Can you work these out from the model? Positions are in its coordinate system, mm. A direction names the side the tool comes from. Round coordinates to 2 decimals unless told otherwise and drop trailing zeros. Loops run counter-clockwise (first coordinate to the right, second up) from the corner with the lowest first, then second, coordinate; pieces in that order, holes last. Notation, with made-up numbers: M -38,48 L -10,48 A26 cw -10,66 Z; hole C 30.25,80 d1. An arc over 180 degrees is marked long. Return JSON: item names as keys, results as strings.
```python
from build123d import *

# Parameters (mm, degrees)
SKETCH3_W            = 88.9
SKETCH3_H            = 88.9
BOSS_EXTRUDE2_DEPTH  = 50.8
SKETCH13_R           = 4.25
CUT_EXTRUDE4_DEPTH   = 102
SKETCH30_W           = 88.9
SKETCH30_H           = 88.9
SKETCH30_W_2         = 60
SKETCH30_H_2         = 60
BOSS_EXTRUDE8_DEPTH  = 110
SKETCH31_W           = 15
SKETCH31_H           = 15
SKETCH31_R           = 2.75
BOSS_EXTRUDE10_DEPTH = 10
FILLET1_R            = 10
SKETCH33_W           = 60
SKETCH33_H           = 60
CUT_EXTRUDE5_DEPTH   = 20
SKETCH37_R           = 2.25
CUT_EXTRUDE6_DEPTH   = 113
SKETCH38_W           = 88.9
SKETCH38_H           = 88.9
CUT_EXTRUDE7_DEPTH   = 41
SKETCH39_W           = 29.45
SKETCH39_H           = 20
BOSS_EXTRUDE11_DEPTH = 20
SKETCH40_W           = 29.45
SKETCH40_H           = 20
BOSS_EXTRUDE12_DEPTH = 20
SKETCH41_R           = 4.25
CUT_EXTRUDE8_DEPTH   = 20
FILLET2_R            = 5
FILLET3_R            = 5


with BuildPart() as part:
    # Sketch3 → Boss-Extrude2 (new body)
    with BuildSketch(Plane(origin=(0, 0, 0), x_dir=(1, 0, 0), z_dir=(0, 1, 0))):
        with Locations((44.45, 44.45)):
            Rectangle(SKETCH3_W, SKETCH3_H)
    extrude(amount=BOSS_EXTRUDE2_DEPTH)

    # Sketch13 → Cut-Extrude4 (cut)
    with BuildSketch(Plane.XY):
        with Locations((44.45, 20)):
            Circle(SKETCH13_R)
    extrude(amount=-CUT_EXTRUDE4_DEPTH, mode=Mode.SUBTRACT)

    # Sketch30 → Boss-Extrude8 (add)
    with BuildSketch(Plane(origin=(0, 50.8, 0), x_dir=(1, 0, 0), z_dir=(0, 1, 0))):
        with Locations((44.45, 44.45)):
            Rectangle(SKETCH30_W, SKETCH30_H)
        with Locations((44.45, 44.45)):
            Rectangle(SKETCH30_W_2, SKETCH30_H_2, mode=Mode.SUBTRACT)
    extrude(amount=BOSS_EXTRUDE8_DEPTH)

    # Sketch31 → Boss-Extrude10 (add)
    # profile 1 of 4: a face of its own
    with BuildSketch(Plane(origin=(0, 160.8, 0), x_dir=(1, 0, 0), z_dir=(0, 1, 0))):
        with Locations((-7.5, 51.95)):
            Rectangle(SKETCH31_W, SKETCH31_H)
        with Locations(Location((-7.5, 51.95, 0), (0, 0, 270))):
            Circle(SKETCH31_R, mode=Mode.SUBTRACT)
    # profile 2 of 4: a face of its own
    with BuildSketch(Plane(origin=(0, 160.8, 0), x_dir=(1, 0, 0), z_dir=(0, 1, 0))):
        with Locations((-7.5, 36.95)):
            Rectangle(SKETCH31_W, SKETCH31_H)
        with Locations(Location((-7.5, 36.95, 0), (0, 0, 270))):
            Circle(SKETCH31_R, mode=Mode.SUBTRACT)
    # profile 3 of 4: a face of its own
    with BuildSketch(Plane(origin=(0, 160.8, 0), x_dir=(1, 0, 0), z_dir=(0, 1, 0))):
        with Locations((96.4, 51.95)):
            Rectangle(SKETCH31_W, SKETCH31_H)
        with Locations(Location((96.4, 51.95, 0), (0, 0, 270))):
            Circle(SKETCH31_R, mode=Mode.SUBTRACT)
    # profile 4 of 4: a face of its own
    with BuildSketch(Plane(origin=(0, 160.8, 0), x_dir=(1, 0, 0), z_dir=(0, 1, 0))):
        with Locations((96.4, 36.95)):
            Rectangle(SKETCH31_W, SKETCH31_H)
        with Locations(Location((96.4, 36.95, 0), (0, 0, 270))):
            Circle(SKETCH31_R, mode=Mode.SUBTRACT)
    extrude(amount=-BOSS_EXTRUDE10_DEPTH)

    # Fillet1
    fillet1_edges = [part.edges().sort_by_distance(p)[0] for p in [
        (0, 80.4, -88.9),
        (88.9, 80.4, -88.9),
        (88.9, 80.4, 0),
        (0, 80.4, 0),
    ]]
    fillet(fillet1_edges, radius=FILLET1_R)

    # Sketch33 → Cut-Extrude5 (cut)
    with BuildSketch(Plane(origin=(88.9, 0, 0), x_dir=(0, 0, -1), z_dir=(1, 0, 0))):
        with Locations((44.45, 80.8)):
            Rectangle(SKETCH33_W, SKETCH33_H)
    extrude(amount=-CUT_EXTRUDE5_DEPTH, mode=Mode.SUBTRACT)

    # Sketch37 → Cut-Extrude6 (cut)
    with BuildSketch(Plane.XY):
        with Locations((81.675, 80.4)):
            Circle(SKETCH37_R)
        with Locations((81.675, 58.4)):
            Circle(SKETCH37_R)
    extrude(amount=-CUT_EXTRUDE6_DEPTH, mode=Mode.SUBTRACT)

    # Sketch38 → Cut-Extrude7 (cut)
    with BuildSketch(Plane.XZ):
        with Locations((44.45, -44.45)):
            Rectangle(SKETCH38_W, SKETCH38_H)
    extrude(amount=-CUT_EXTRUDE7_DEPTH, mode=Mode.SUBTRACT)

    # Sketch39 → Boss-Extrude11 (add)
    with BuildSketch(Plane.XY):
        with Locations((29.725, 51)):
            Rectangle(SKETCH39_W, SKETCH39_H)
        with Locations((59.175, 51)):
            Rectangle(SKETCH39_W, SKETCH39_H)
    extrude(amount=BOSS_EXTRUDE11_DEPTH)

    # Sketch40 → Boss-Extrude12 (add)
    with BuildSketch(Plane(origin=(0, 0, -88.9), x_dir=(-1, 0, 0), z_dir=(0, 0, -1))):
        with Locations((-59.175, 51)):
            Rectangle(SKETCH40_W, SKETCH40_H)
        with Locations((-29.725, 51)):
            Rectangle(SKETCH40_W, SKETCH40_H)
    extrude(amount=BOSS_EXTRUDE12_DEPTH)

    # Sketch41 → Cut-Extrude8 (cut)
    with BuildSketch(Plane.XZ.offset(-41)):
        with Locations(Location((63.9, 10, 0), (0, 0, 270))):
            Circle(SKETCH41_R)
        with Locations(Location((25, 10, 0), (0, 0, 270))):
            Circle(SKETCH41_R)
        with Locations(Location((63.9, -98.9, 0), (0, 0, 270))):
            Circle(SKETCH41_R)
        with Locations(Location((25, -98.9, 0), (0, 0, 270))):
            Circle(SKETCH41_R)
    extrude(amount=-CUT_EXTRUDE8_DEPTH, mode=Mode.SUBTRACT)

    # Fillet2
    fillet2_edges = [part.edges().sort_by_distance(p)[0] for p in [
        (15, 51, -108.9),
        (15, 51, -88.9),
        (73.9, 51, -108.9),
        (73.9, 51, -88.9),
        (73.9, 51, 0),
        (15, 51, 0),
        (15, 51, 20),
        (73.9, 51, 20),
    ]]
    fillet(fillet2_edges, radius=FILLET2_R - 0.0001)  # a hair under: the kernel refuses the full size

    # Fillet3
    fillet3_edges = [part.edges().sort_by_distance(p)[0] for p in [
        (-15, 155.8, -29.45),
        (-15, 155.8, -59.45),
        (0, 155.8, -59.45),
        (0, 155.8, -29.45),
        (88.9, 155.8, -29.45),
        (88.9, 155.8, -59.45),
        (103.9, 155.8, -59.45),
        (103.9, 155.8, -29.45),
    ]]
    fillet(fillet3_edges, radius=FILLET3_R)


solid = part.part
```
Q1. Suppose I cut it at C-C, the plane z = -51.95. Please give me the cut outline in (x, y).
Results:
{"outline": "M -15,150.8 L -10.25,150.8 L -10.25,160.8 L -15,160.8 Z; M -4.75,150.8 L 0,150.8 L 0,41 L 88.9,41 L 88.9,50.8 L 14.45,50.8 L 14.45,160.8 L -4.75,160.8 Z; M 74.45,110.8 L 88.9,110.8 L 88.9,150.8 L 93.65,150.8 L 93.65,160.8 L 74.45,160.8 Z; M 99.15,150.8 L 103.9,150.8 L 103.9,160.8 L 99.15,160.8 Z"}
Q2. If I drill on line 1 along X through (y, z) = (52, -99); line 2 along Z through (x, y) = (46.5, 134); line 3 along X through (y, z) = (55, -95), over which ranges is the centre line in solid material (lowest first)?
Results:
{"line 1": "x = 15 to 20.75, 29.25 to 59.65, 68.15 to 73.9", "line 2": "z = -88.9 to -74.45, -14.45 to 0", "line 3": "x = 15 to 23.31, 26.69 to 62.21, 65.59 to 73.9"}
Q3. Suppose I cut it at B-B, the plane z = 10. Please give me the cut outline in (x, y), plus the area to 3 significant figures.
Results:
{"outline": "M 15,41 L 20.75,41 L 20.75,61 L 15,61 Z; M 29.25,41 L 59.65,41 L 59.65,61 L 29.25,61 Z; M 68.15,41 L 73.9,41 L 73.9,61 L 68.15,61 Z", "area": "838 mm2"}
Q4. I'm going to push flat-ended pins straight in: pin 1 Ø5 at (x, y) = (86, 124.5) entering from -Z; pin 2 Ø6 at (x, y) = (69.5, 82.5) entering from +Z; pin 3 Ø5 at (y, z) = (90, -90.5) entering from +X; pin 4 Ø3.5 at (x, y) = (81.675, 58.4) entering from +Z. Where does each tip first touch, or does it pass through?
Results:
{"pin 1": "stops at z = -87.78", "pin 2": "stops at z = 0", "pin 3": "stops at x = 83.05", "pin 4": "passes through"}
Q5. Suppose I cut it at A-A, the plane x = 25. Please give me the cut outline in (y, z), plus the area to 3 significant figures.
Results:
{"outline": "M 41,-108.9 L 61,-108.9 L 61,-103.15 L 41,-103.15 Z; M 41,-94.65 L 61,-94.65 L 61,-88.9 L 160.8,-88.9 L 160.8,-74.45 L 50.8,-74.45 L 50.8,-14.45 L 160.8,-14.45 L 160.8,0 L 61,0 L 61,5.75 L 41,5.75 Z; M 41,14.25 L 61,14.25 L 61,20 L 41,20 Z", "area": "4,510 mm2"}
Q6. On a 3-axis mill with a long thin cutter (end or side, diameter ignored), from which of +Z, -Z, +X, -X, +Y, -Y can I reach the whole of each face in a straight line? I mean faces 4 (the flat face through (44, 113, 0)), 5 (the flat face through (15, 51, -99)), 6 (the flat face through (-8, 156, -29.45)), 7 (the flat face through (52, 50.8, -44)). Say none if no direction works.
Results:
{"face 4": "+Z, +X, -X, +Y", "face 5": "-Z, -X, +Y, -Y", "face 6": "+Z, -X, +Y, -Y", "face 7": "+X"}
Q7. Thinking about a two-plate mould opening in X: for faces 1 (the cylindrical face through (26.277, 50.86, 5.946)), 2 (the cylindrical face through (16.43, 51.14, -107.4)), 3 (the cylindrical face through (86.05, 101.74, -3.01)), which applies, pulls with the +X half, pulls with the -X half, needs draft (parallel to the pull), parting line crosses it, or undercut?
Results:
{"face 1": "undercut", "face 2": "pulls with the -X half", "face 3": "pulls with the +X half"}
Q8. Suppose I cut it at D-D, the plane y = 84.5. Please give me the cut outline in (x, z).
Results:
{"outline": "M 0,-78.9 A10 ccw 10,-88.9 L 78.9,-88.9 A10 ccw 88.9,-78.9 L 88.9,-74.45 L 14.45,-74.45 L 14.45,-14.45 L 88.9,-14.45 L 88.9,-10 A10 ccw 78.9,0 L 10,0 A10 ccw 0,-10 Z"}
